Geometry: final body of the model. Coordinates: model frame, mm. A direction names the side the tool comes from. Round coordinates to 2 decimals unless told otherwise and drop trailing zeros. Order: outer loops, then holes, each group sorted by start corner. A loop starts at its lowest first (then second) coordinate and runs counter-clockwise, first axis right, second up. Notation, with made-up numbers: (-21, 42.25) -> (-9, 42.25) arc R20 ccw to (-9, 50.25) -> close; hole circle Ø11 at (45.5, 54). An arc over 180 degrees is marked (long way). Put each result on its own line as item: value.
```python
from build123d import *

# Parameters (mm, degrees)
F0_W      = 96
F0_H      = 54
F1_DEPTH  = 25
F2_SIZE2  = 35
F2_SIZE   = 18
F4_DEPTH  = 50.001
F5_R      = 20
F6_DEPTH  = 30
F7_W      = 40
F7_H      = 16
F8_DEPTH  = 20
F9_W      = 30
F9_H      = 28
F10_DEPTH = 23


# Not quite as in the source:
# - a pattern or mirror of a feature is missing from the dataset's text; its kind, count and spacing are read off the source's solid


with BuildPart() as f1:
    # F0 (on Right) → F1 (new body, symmetric)
    with BuildSketch(Plane.YZ):
        Rectangle(F0_W, F0_H)
    extrude(amount=F1_DEPTH, both=True)

    # F2
    f2_edges = [f1.edges().sort_by_distance(p)[0] for p in [
        (0, -48, 27),
        (0, 48, 27),
    ]]
    f2_side = f1.faces().sort_by_distance((0, 0, 27))[0]
    chamfer(f2_edges, length=F2_SIZE, length2=F2_SIZE2, reference=f2_side)

    # F3 (on face) → F4 (cut, through all)
    with BuildSketch(Plane.YZ.offset(25)):
        Polygon((-10, -7), (-20, -27), (20, -27), (10, -7), align=None)
    extrude(amount=-F4_DEPTH, mode=Mode.SUBTRACT)

    # F5 (on face) → F6 (join)
    with BuildSketch(Plane.XY.offset(27)):
        Circle(F5_R)
    extrude(amount=F6_DEPTH)

    # F7 (on face) → F8 (cut)
    with BuildSketch(Plane.XY.offset(57)):
        Rectangle(F7_W, F7_H)
    extrude(amount=-F8_DEPTH, mode=Mode.SUBTRACT)

    # F9 (on face) → F10 (cut)
    with BuildSketch(Plane.XZ.offset(48)):
        with Locations((0, 13)):
            Rectangle(F9_W, F9_H)
    f10 = extrude(amount=-F10_DEPTH, mode=Mode.SUBTRACT)

    # F10_copies: F10 across plane
    add(f10.mirror(Plane.ZX), mode=Mode.SUBTRACT)


solid = f1.part
```
1. Material intervals for probe 1 along X at (y, z) = (-27, 24.5); probe 2 along Y at (x, z) = (-13.5, 23); probe 3 along Y at (x, z) = (4.5, -17), sorted ascending.
Ans:
probe 1: -25 to -15, 15 to 25
probe 2: -25 to 25
probe 3: -48 to -15, 15 to 48
2. Contact query for flat-ended pins moving along their axis: P1, Ø6, axis at x = 4.5, y = 1, coming from the -Z side; P2, Ø10, axis at x = 7.5, z = 43, coming from the +Y side; P3, Ø2, axis at y = -16, z = 36.5, coming from the +X side. Output: stop coordinate, or through.
Ans:
P1: z = -7
P2: y = 19.84
P3: x = 13.23
3. Cut plane C-C on x = 12. Return loops of the section in (y, z), and give its area (3 significant figures).
Ans:
outline: (-48, -27) -> (-20, -27) -> (-10, -7) -> (10, -7) -> (20, -27) -> (48, -27) -> (48, -8) -> (44.4, -1) -> (25, -1) -> (25, 27) -> (16, 27) -> (16, 57) -> (8, 57) -> (8, 37) -> (-8, 37) -> (-8, 57) -> (-16, 57) -> (-16, 27) -> (-25, 27) -> (-25, -1) -> (-44.4, -1) -> (-48, -8) -> close
area: 3,910 mm²
4. Cut plane B-B on y = -39. Return loops of the section in (x, z), and give its area (3 significant figures).
Ans:
outline: (-25, -27) -> (25, -27) -> (25, 9.5) -> (15, 9.5) -> (15, -1) -> (-15, -1) -> (-15, 9.5) -> (-25, 9.5) -> close
area: 1,510 mm²
5. Draft query along X for faces 5 (the face through (0, 13, 57)), 6 (the face through (0, 35, -1)), 7 (the face through (-16, -12, 42)). Return one class per face: +X half, -X half, draft (parallel to the pull), parting line (faces both ways), or undercut.
Ans:
face 5: draft
face 6: undercut
face 7: parting line
6. Cut plane D-D on z = 4. Return loops of the section in (x, y).
Ans:
outline: (-25, -41.83) -> (-15, -41.83) -> (-15, -25) -> (15, -25) -> (15, -41.83) -> (25, -41.83) -> (25, 41.83) -> (15, 41.83) -> (15, 25) -> (-15, 25) -> (-15, 41.83) -> (-25, 41.83) -> close
7. Set-up query: faces 1 (the face through (15, -33, 10)), 2 (the face through (15, 33, 10)), 3 (the face through (0, 0, 37)), 4 (the face through (0, 0, -7)). Return all of +Z, -Z, +X, -X, +Y, -Y with unobstructed straight access to the full face (end or side cutting, diameter ignored); none if empty.
Ans:
face 1: +Z, -Y
face 2: +Z, +Y
face 3: +Z, +X, -X
face 4: -Z, +X, -X
8. Cut plane A-A on z = -18. Return loops of the section in (x, y).
Ans:
outline: (-25, -48) -> (25, -48) -> (25, -15.5) -> (-25, -15.5) -> close; (-25, 15.5) -> (25, 15.5) -> (25, 48) -> (-25, 48) -> close
